The model under review builds one solid part; all positions refer to its coordinate system, in mm. Round coordinates to 2 decimals unless told otherwise and drop trailing zeros. Write each loop counter-clockwise with the first axis right and the second up, starting at its lowest first coordinate (ties: lowest second). Pieces come first, ordered by that corner, then holes. Notation, with made-up numbers: (83, 48.5) -> (91, 48.5) arc R27 cw to (91, 79.5) -> close; hole circle Ø4 at (88.5, 88.25). An arc over 180 degrees is marked (long way). Answer as a JSON object with one key per item and string values. Group by question number.
1) Insertion check: pin 1 Ø0.8 at (y, z) = (2, 1) entering from +X; pin 2 Ø1 at (x, y) = (16.5, 19) entering from -Z. Each pin has a flat end and moves straight along its axis. Give the tip position at first contact, or say it passes through.
2) We need section A-A, the plane z = 0.35. Write out the cut boundary in (x, y).
3) We need section C-C, the plane y = 49.5. Write out the cut boundary in (x, z), then the cut area to 3 significant figures.
4) We need section B-B, the plane x = 17.5. Write out the cut boundary in (y, z).
5) To check wall thickness, follow probe 1 along Y at (x, z) = (17, 0.9); probe 2 along X at (y, z) = (45.5, 0.9); probe 3 along Y at (x, z) = (26, 0.6). State the ranges of each line that lie inside material, in increasing order. Write a range as [from, to].
6) We need section D-D, the plane y = 25. Write out the cut boundary in (x, z).
from build123d import *

# Parameters (mm, degrees)
SKIZZE1_W                       = 35
SKIZZE1_H                       = 75
AUFSATZ_LINEAR_AUSTRAGEN1_DEPTH = 1.5
SKIZZE2_W                       = 11.63
SKIZZE2_H                       = 5
SKIZZE2_W_2                     = 11.62
SKIZZE2_W_3                     = 1.75
SCHNITT_LINEAR_AUSTRAGEN1_DEPTH = 1.5
SCHNITT_LINEAR_AUSTRAGEN5_DEPTH = 20
SCHNITT_LINEAR_AUSTRAGEN6_DEPTH = 20


with BuildPart() as part:
    # Skizze1 → Aufsatz-Linear austragen1 (new body)
    with BuildSketch(Plane.XY):
        with Locations((17.5, 37.5)):
            Rectangle(SKIZZE1_W, SKIZZE1_H)
    extrude(amount=AUFSATZ_LINEAR_AUSTRAGEN1_DEPTH)

    # Skizze2 → Schnitt-Linear austragen1 (cut)
    with BuildSketch(Plane.XY.offset(1.5)):
        with Locations((5.815, 2.5)):
            Rectangle(SKIZZE2_W, SKIZZE2_H)
        with Locations((29.19, 2.5)):
            Rectangle(SKIZZE2_W_2, SKIZZE2_H)
        with Locations((17.505, 2.5)):
            Rectangle(SKIZZE2_W_3, SKIZZE2_H)
    extrude(amount=-SCHNITT_LINEAR_AUSTRAGEN1_DEPTH, mode=Mode.SUBTRACT)

    # Skizze10 → Schnitt-Linear austragen5 (cut)
    with BuildSketch(Plane.XY.offset(1.5)):
        with BuildLine():
            Line((7.35039959, 38.082998074), (6.35039959, 38.370002144))
            ThreePointArc((6.35039959, 38.370002144), (30.439070096, 32.099486097), (6.902625657, 23.998918129))
            Line((6.902625657, 23.998918129), (8.1632503, 23.998918129))
            ThreePointArc((8.1632503, 23.998918129), (29.428721451, 32.291733198), (7.35039959, 38.082998074))
        make_face()
    extrude(amount=-SCHNITT_LINEAR_AUSTRAGEN5_DEPTH, mode=Mode.SUBTRACT)

    # Skizze11 → Schnitt-Linear austragen6 (cut)
    with BuildSketch(Plane.XY.offset(1.5)):
        Polygon((7.35039959, 38.082998074), (6.35039959, 38.082998074), (6.35039959, 64.5), (7.35039959, 64.5), (28.25, 64.5), (28.25, 63.5), (7.35039959, 63.5), align=None)
    extrude(amount=-SCHNITT_LINEAR_AUSTRAGEN6_DEPTH, mode=Mode.SUBTRACT)


solid = part.part
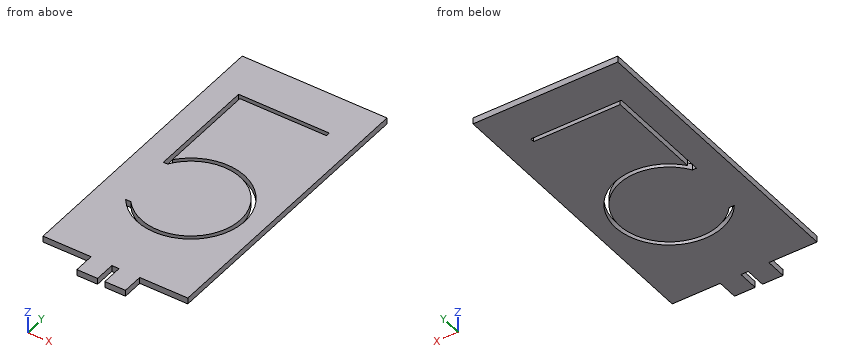
Here are the results:
{
 "1": {"pin 1": "stops at x = 23.38", "pin 2": "stops at z = 0"},
 "2": {"outline": "(0, 5) -> (11.63, 5) -> (11.63, 0) -> (16.63, 0) -> (16.63, 5) -> (18.38, 5) -> (18.38, 0) -> (23.38, 0) -> (23.38, 5) -> (35, 5) -> (35, 75) -> (0, 75) -> close; hole (6.35, 38.08) -> (7.35, 38.08) arc R12 cw (long way) to (8.16, 24) -> (6.9, 24) arc R13 ccw (long way) to (7.35, 39.79) -> (7.35, 63.5) -> (28.25, 63.5) -> (28.25, 64.5) -> (6.35, 64.5) -> close"},
 "3": {"outline": "(0, 0) -> (6.35, 0) -> (6.35, 1.5) -> (0, 1.5) -> close; (7.35, 0) -> (35, 0) -> (35, 1.5) -> (7.35, 1.5) -> close", "area": "51.0 mm^2"},
 "4": {"outline": "(5, 0) -> (18.6, 0) -> (18.6, 1.5) -> (5, 1.5) -> close; (19.6, 0) -> (43.6, 0) -> (43.6, 1.5) -> (19.6, 1.5) -> close; (44.6, 0) -> (63.5, 0) -> (63.5, 1.5) -> (44.6, 1.5) -> close; (64.5, 0) -> (75, 0) -> (75, 1.5) -> (64.5, 1.5) -> close"},
 "5": {"probe 1": "y = [5, 18.61], [19.61, 43.59], [44.59, 63.5], [64.5, 75]", "probe 2": "x = [0, 6.35], [7.35, 35]", "probe 3": "y = [5, 21.81], [23.18, 40.02], [41.39, 63.5], [64.5, 75]"},
 "6": {"outline": "(0, 0) -> (27.47, 0) -> (27.47, 1.5) -> (0, 1.5) -> close; (28.65, 0) -> (35, 0) -> (35, 1.5) -> (28.65, 1.5) -> close"}
}
